```python
from build123d import *

# Parameters (mm, degrees)
EXTRUDE_1_DEPTH              = 31.5
HOLE_WIZARD_M3_1_D           = 2.5
HOLE_WIZARD_M3_1_DEPTH       = 14
HOLE_WIZARD_M3_1_CBORE_D     = 3
HOLE_WIZARD_M3_1_CBORE_DEPTH = 13.5
HOLE_WIZARD_M3_1_TIP         = 0.751075774
HOLE_WIZARD_M4_1_D           = 4.3
CUT_EXTRUDE_1_REACH          = 54.012
SKETCH_6_W                   = 55
SKETCH_6_H                   = 6.3
CHAMFER_1_SIZE               = 1


with BuildPart() as part:
    # 草图1 → 凸台-拉伸1 (new, symmetric)
    with BuildSketch(Plane.XY):
        Polygon((-27.5, 19.1), (-38, 19.1), (-38, 0), (38, 0), (38, 19.1), (27.5, 19.1), (27.5, 13.3), (31.6, 13.3), (31.6, 2.7), (-31.6, 2.7), (-31.6, 13.3), (-27.5, 13.3), align=None)
    extrude(amount=EXTRUDE_1_DEPTH, both=True)

    # M3 螺纹孔1
    with Locations(Plane(origin=(0, 0, 0), x_dir=(-1, 0, 0), z_dir=(0, -1, 0))):
        with Locations((34.8, 25.5), (34.8, -25.5), (-34.8, -25.5), (-34.8, 25.5)):
            CounterBoreHole(HOLE_WIZARD_M3_1_D / 2, HOLE_WIZARD_M3_1_CBORE_D / 2, HOLE_WIZARD_M3_1_CBORE_DEPTH, depth=HOLE_WIZARD_M3_1_DEPTH)
            with Locations((0, 0, -(HOLE_WIZARD_M3_1_DEPTH + HOLE_WIZARD_M3_1_TIP / 2))):  # 118° drill point
                Cone(0, HOLE_WIZARD_M3_1_D / 2, HOLE_WIZARD_M3_1_TIP, mode=Mode.SUBTRACT)

    # M4 间隙孔1 (through all)
    with Locations(Plane(origin=(0, 0, 0), x_dir=(-1, 0, 0), z_dir=(0, -1, 0))):
        with Locations((-14, 12.2), (14, 12.2)):
            Hole(HOLE_WIZARD_M4_1_D / 2)

    # 草图6 → 切除-拉伸1 (cut, up to next)
    with BuildSketch(Plane(origin=(0, 2.7, 0), x_dir=(1, 0, 0), z_dir=(0, 1, 0)), mode=Mode.PRIVATE) as cut_extrude_1_sk1:
        with Locations((0, 28.35)):
            Rectangle(SKETCH_6_W, SKETCH_6_H)
    cut_extrude_1_tool1 = extrude(cut_extrude_1_sk1.sketch, amount=-CUT_EXTRUDE_1_REACH, mode=Mode.PRIVATE) & part.part
    add(cut_extrude_1_tool1.solids().sort_by_distance((0, 2.7, -28.35))[0], mode=Mode.SUBTRACT)

    # 倒角1
    chamfer_1_edges = [part.edges().sort_by_distance(p)[0] for p in [
        (-27.5, 13.3, 0),
        (27.5, 13.3, 0),
        (27.5, 19.1, 0),
        (-27.5, 19.1, 0),
    ]]
    chamfer(chamfer_1_edges, length=CHAMFER_1_SIZE)


solid = part.part
```
The model under review builds one solid part; all positions refer to its coordinate system, in mm. A direction names the side the tool comes from. Give positions to 0.01 mm unless a question says otherwise; leave off trailing zeros. Write each loop counter-clockwise with the first axis right and the second up, starting at its lowest first coordinate (ties: lowest second). Pieces come first, ordered by that corner, then holes. Notation, with made-up numbers: M -16,11 L 6,11 A25 cw 6,26 Z; hole C 3.5,31 d10. An arc over 180 degrees is marked long. Write item = value, one per line. Start each with the question number.
Q1. We need section B-B (z = -12.2). State the section outline as (x, y) points, plus the area to 3 significant figures.
Q2. Machinability: for faces 4 (the face through (31.6, 8, 0)), 5 (the face through (-27.5, 16, 0)), 6 (the face through (35.91, 6.66, -26.51)), which of the approach directions +Z, -Z, +X, -X, +Y, -Y give a long, thin tool a straight path to every point of the face, cutting with its end or side? Answer none if there is none.
Q3. Mouldability with a two-part tool opening along Z and no side actions: class faces 1 (the face through (0, 1, -25.2)), 2 (the face through (-35.01, 14.62, -25.57)), 3 (the face through (-38, 10, 0)) as released by +Z, released by -Z, zero draft, split by the parting line, or undercut.
Q4. We need section A-A (y = 6.25). State the section outline as (x, z) points.
Q5. For line 1 (Z direction, x = -34.8, y = 13.75); line 2 (X direction, y = 1.3, z = -12.2); line 3 (X direction, y = 4.25, z = 25.5), list the stretches that pass through material, from the lowest coordinate up.
Q6. Clearance check with flat-ended pins moving along their axes: pin 1 (0.9 mm diameter, centred on x = -35.5, z = 25.5, fed in from -Y); pin 2 (3 mm diameter, centred on x = 9.5, y = 1.5, fed in from -Z); pin 3 (1.5 mm diameter, centred on x = -34.8, z = 25.5, fed in from -Y). State where each tip first meets the part, or that it passes through.
Q7. We need section D-D (y = 17). State the section outline as (x, z) points.
Q8. We need section C-C (x = -14). State the section outline as (y, z) points, plus the area to 3 significant figures.
Result set:
q1.outline = M -38,0 L -16.15,0 L -16.15,2.7 L -31.6,2.7 L -31.6,13.3 L -28.5,13.3 L -27.5,14.3 L -27.5,18.1 L -28.5,19.1 L -38,19.1 Z; M -11.85,0 L 11.85,0 L 11.85,2.7 L -11.85,2.7 Z; M 16.15,0 L 38,0 L 38,19.1 L 28.5,19.1 L 27.5,18.1 L 27.5,14.3 L 28.5,13.3 L 31.6,13.3 L 31.6,2.7 L 16.15,2.7 Z
q1.area = 437 mm2
q2.face_4 = +Z, -Z
q2.face_5 = +Z, -Z, +Y
q2.face_6 = -Y
q3.face_1 = released by -Z
q3.face_2 = undercut
q3.face_3 = zero draft
q4.outline = M -38,-31.5 L -31.6,-31.5 L -31.6,31.5 L -38,31.5 Z; M 31.6,-31.5 L 38,-31.5 L 38,31.5 L 31.6,31.5 Z; hole C -34.8,-25.5 d3; hole C -34.8,25.5 d3; hole C 34.8,-25.5 d3; hole C 34.8,25.5 d3
q5.line_1 = -31.5 to -26.75, -24.25 to 24.25, 26.75 to 31.5
q5.line_2 = -38 to -16.15, -11.85 to 11.85, 16.15 to 38
q5.line_3 = -38 to -36.3, -33.3 to -31.6, 31.6 to 33.3, 36.3 to 38
q6.pin_1 = 14.06
q6.pin_2 = -25.2
q6.pin_3 = 14.3
q7.outline = M -38,-31.5 L -27.5,-31.5 L -27.5,31.5 L -38,31.5 Z; M 27.5,-31.5 L 38,-31.5 L 38,31.5 L 27.5,31.5 Z
q8.outline = M 0,-25.2 L 2.7,-25.2 L 2.7,-14.35 L 0,-14.35 Z; M 0,-10.05 L 2.7,-10.05 L 2.7,31.5 L 0,31.5 Z
q8.area = 141 mm2
